Study the drawing (mm; zero at the part's minimum x, y, z) and answer. A direction names the side the tool comes from. Coordinates: 2 decimals unless noted, no trailing zeros. Write each loop counter-clockwise with the first axis right and the second up, starting at its lowest first coordinate (ties: lowest second). Pieces come first, ordered by that corner, then holes. Notation, with made-up numbers: M -30,-37.75 L 8,-37.75 A11 ccw 8,-24.75 Z; hole C 88,25.25 d10. An arc over 180 degrees is marked long. Answer as CSV lines item,"result". Start each with the question number.
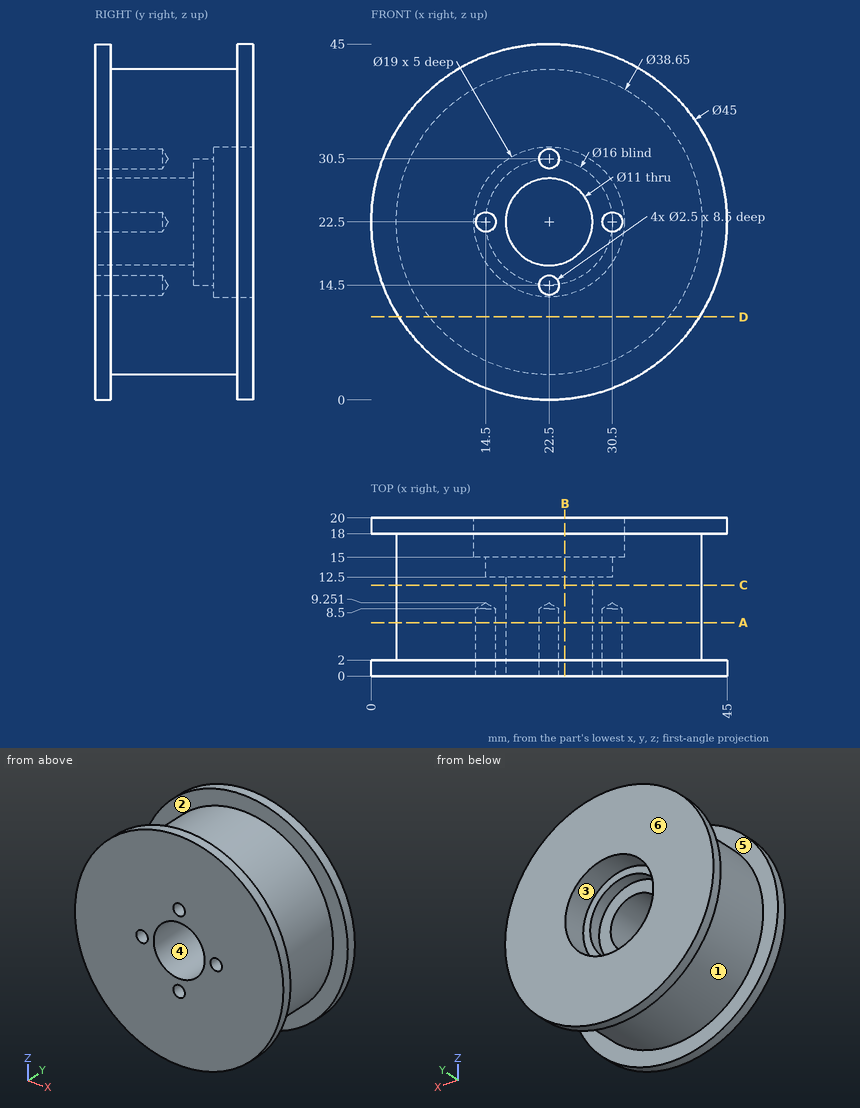
1) The part is cut by section C-C (y = 11.5). Determine the outline of the cut face in (x, z) (3 decimals).
2) The part is cut by section D-D (z = 10.5). Determine the outline of the cut face in (x, y), then the cut area to 3 significant figures.
3) Which of the six approach directions +Z, -Z, +X, -X, +Y, -Y give full straight-line access (tool end or side, diameter ignored) to the marked faces 5 and 6?
4) Each of these flat-tipped pins is pushed along its axis until it touches: P1, Ø12, axis at y = 11, z = 33, coming from the -X side; P2, Ø4, axis at y = 8, z = 15.5, coming from the +X side; P3, Ø18.5, axis at x = 22.5, z = 22.5, coming from the +Y side; P4, Ø17.5, axis at x = 19, z = 23, coming from the +Y side. Where does it stop, or does it pass through?
5) The part is cut by section A-A (y = 6.75). Determine the outline of the cut face in (x, z) (3 decimals), then the cut area to 3 significant figures.
6) For a pull along Z with two mould halves and no side action, classify the marked faces 1, 2, 3 and 4 as +Z half, -Z half, draft (parallel to the pull), parting line (faces both ways), or undercut.
7) Find the intervals of material crossed by line 1 (X direction, y = 17.5, z = 22.5) (3 decimals); line 2 (Z direction, x = 22.5, y = 2.5) (3 decimals); line 3 (Y direction, x = 37.5, z = 8.5), in increasing order. Write a range as from..to.
8) The part is cut by section B-B (x = 24.5). Determine the outline of the cut face in (y, z), then the cut area to 3 significant figures.
Completed:
1,outline,"C 22.5,22.5 d38.65; hole C 22.5,22.5 d11"
2,outline,"M 3.47,0 L 41.53,0 L 41.53,2 L 37.65,2 L 37.65,18 L 41.53,18 L 41.53,20 L 3.47,20 L 3.47,18 L 7.35,18 L 7.35,2 L 3.47,2 Z"
2,area,"637 mm²"
3,face 5,"none"
3,face 6,"+Z, -Z, +X, -X, +Y"
4,P1,"x = 3.71"
4,P2,"x = 41.17"
4,P3,"y = 15"
4,P4,"y = 20"
5,outline,"C 22.5,22.5 d38.65; hole C 14.5,22.5 d2.5; hole C 22.5,22.5 d11; hole C 22.5,14.5 d2.5; hole C 22.5,30.5 d2.5; hole C 30.5,22.5 d2.5"
5,area,"1,060 mm²"
6,face 1,"parting line"
6,face 2,"draft"
6,face 3,"undercut"
6,face 4,"undercut"
7,line 1,"3.175..13, 32..41.825"
7,line 2,"3.175..13.25, 15.75..17, 28..29.25, 31.75..41.825"
7,line 3,"0..2, 18..20"
8,outline,"M 0,0.09 L 2,0.09 L 2,3.28 L 18,3.28 L 18,0.09 L 20,0.09 L 20,13.21 L 15,13.21 L 15,14.75 L 12.5,14.75 L 12.5,17.38 L 0,17.38 Z; M 0,27.62 L 12.5,27.62 L 12.5,30.25 L 15,30.25 L 15,31.79 L 20,31.79 L 20,44.91 L 18,44.91 L 18,41.72 L 2,41.72 L 2,44.91 L 0,44.91 Z"
8,area,"535 mm²"
